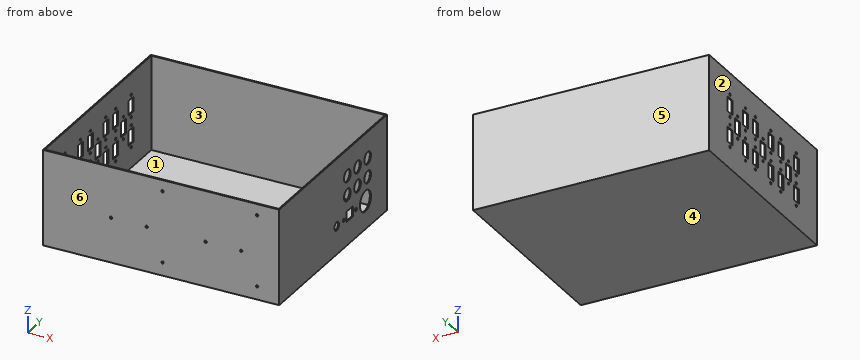
```python
from build123d import *

# Parameters (mm, degrees)
SKETCH2_W                        = 298.45
SKETCH2_H                        = 254
BOSS_EXTRUDE1_DEPTH              = 120.65
SHELL1_T                         = -1.5
PT_CONNECTOR_CUTOUTS_REACH       = 348.06
SKETCH3_R                        = 7.8105
SKETCH3_R_2                      = 2.06375
SKETCH3_R_3                      = 5.334
SKETCH3_R_4                      = 13.0175
SKETCH3_W                        = 13.081
SKETCH3_H                        = 15.748
SKETCH4_R                        = 1.55
SKETCH4_W                        = 18.7
SKETCH4_H                        = 11.8
SOLENOID_CONNECTOR_CUTOUTS_DEPTH = 1.5
SKETCH5_R                        = 1.524
PCB_MOUNTING_HOLES_DEPTH         = 1.5


with BuildPart() as part:
    # Sketch2 → Boss-Extrude1 (new body)
    with BuildSketch(Plane.XY):
        Rectangle(SKETCH2_W, SKETCH2_H)
    extrude(amount=BOSS_EXTRUDE1_DEPTH)

    # Shell1
    shell1_openings = [part.faces().sort_by_distance(p)[0] for p in [
        (0, 0, 120.65),
    ]]
    offset(amount=SHELL1_T, openings=shell1_openings, kind=Kind.INTERSECTION)

    # Sketch3 → PT Connector Cutouts (cut, up to next)
    with BuildSketch(Plane(origin=(149.225, 0, 0), x_dir=(0, 0, -1), z_dir=(1, 0, 0)), mode=Mode.PRIVATE) as pt_connector_cutouts_sk1:
        with Locations((-87.4395, 33.555885142)):
            Circle(SKETCH3_R)
    pt_connector_cutouts_tool1 = extrude(pt_connector_cutouts_sk1.sketch, amount=-PT_CONNECTOR_CUTOUTS_REACH, mode=Mode.PRIVATE) & part.part
    # Sketch3 → PT Connector Cutouts (cut, up to next)
    with BuildSketch(Plane(origin=(149.225, 0, 0), x_dir=(0, 0, -1), z_dir=(1, 0, 0)), mode=Mode.PRIVATE) as pt_connector_cutouts_sk2:
        with Locations((-63.4395, 33.555885142)):
            Circle(SKETCH3_R)
    pt_connector_cutouts_tool2 = extrude(pt_connector_cutouts_sk2.sketch, amount=-PT_CONNECTOR_CUTOUTS_REACH, mode=Mode.PRIVATE) & part.part
    # Sketch3 → PT Connector Cutouts (cut, up to next)
    with BuildSketch(Plane(origin=(149.225, 0, 0), x_dir=(0, 0, -1), z_dir=(1, 0, 0)), mode=Mode.PRIVATE) as pt_connector_cutouts_sk3:
        with Locations((-63.4395, 57.555885142)):
            Circle(SKETCH3_R)
    pt_connector_cutouts_tool3 = extrude(pt_connector_cutouts_sk3.sketch, amount=-PT_CONNECTOR_CUTOUTS_REACH, mode=Mode.PRIVATE) & part.part
    # Sketch3 → PT Connector Cutouts (cut, up to next)
    with BuildSketch(Plane(origin=(149.225, 0, 0), x_dir=(0, 0, -1), z_dir=(1, 0, 0)), mode=Mode.PRIVATE) as pt_connector_cutouts_sk4:
        with Locations((-63.4395, 81.555885142)):
            Circle(SKETCH3_R)
    pt_connector_cutouts_tool4 = extrude(pt_connector_cutouts_sk4.sketch, amount=-PT_CONNECTOR_CUTOUTS_REACH, mode=Mode.PRIVATE) & part.part
    # Sketch3 → PT Connector Cutouts (cut, up to next)
    with BuildSketch(Plane(origin=(149.225, 0, 0), x_dir=(0, 0, -1), z_dir=(1, 0, 0)), mode=Mode.PRIVATE) as pt_connector_cutouts_sk5:
        with Locations((-87.4395, 57.555885142)):
            Circle(SKETCH3_R)
    pt_connector_cutouts_tool5 = extrude(pt_connector_cutouts_sk5.sketch, amount=-PT_CONNECTOR_CUTOUTS_REACH, mode=Mode.PRIVATE) & part.part
    # Sketch3 → PT Connector Cutouts (cut, up to next)
    with BuildSketch(Plane(origin=(149.225, 0, 0), x_dir=(0, 0, -1), z_dir=(1, 0, 0)), mode=Mode.PRIVATE) as pt_connector_cutouts_sk6:
        with Locations((-87.4395, 81.555885142)):
            Circle(SKETCH3_R)
    pt_connector_cutouts_tool6 = extrude(pt_connector_cutouts_sk6.sketch, amount=-PT_CONNECTOR_CUTOUTS_REACH, mode=Mode.PRIVATE) & part.part
    # Sketch3 → PT Connector Cutouts (cut, up to next)
    with BuildSketch(Plane(origin=(149.225, 0, 0), x_dir=(0, 0, -1), z_dir=(1, 0, 0)), mode=Mode.PRIVATE) as pt_connector_cutouts_sk7:
        with Locations((-35.418702679, 25.011064362)):
            Circle(SKETCH3_R_2)
    pt_connector_cutouts_tool7 = extrude(pt_connector_cutouts_sk7.sketch, amount=-PT_CONNECTOR_CUTOUTS_REACH, mode=Mode.PRIVATE) & part.part
    # Sketch3 → PT Connector Cutouts (cut, up to next)
    with BuildSketch(Plane(origin=(149.225, 0, 0), x_dir=(0, 0, -1), z_dir=(1, 0, 0)), mode=Mode.PRIVATE) as pt_connector_cutouts_sk8:
        with Locations(Location((-35.418702679, 53.840064362, 0), (0, 0, 180))):
            Circle(SKETCH3_R_2)
    pt_connector_cutouts_tool8 = extrude(pt_connector_cutouts_sk8.sketch, amount=-PT_CONNECTOR_CUTOUTS_REACH, mode=Mode.PRIVATE) & part.part
    # Sketch3 → PT Connector Cutouts (cut, up to next)
    with BuildSketch(Plane(origin=(149.225, 0, 0), x_dir=(0, 0, -1), z_dir=(1, 0, 0)), mode=Mode.PRIVATE) as pt_connector_cutouts_sk9:
        with Locations((-35.56, 8.501064362)):
            Circle(SKETCH3_R_3)
    pt_connector_cutouts_tool9 = extrude(pt_connector_cutouts_sk9.sketch, amount=-PT_CONNECTOR_CUTOUTS_REACH, mode=Mode.PRIVATE) & part.part
    # Sketch3 → PT Connector Cutouts (cut, up to next)
    with BuildSketch(Plane(origin=(149.225, 0, 0), x_dir=(0, 0, -1), z_dir=(1, 0, 0)), mode=Mode.PRIVATE) as pt_connector_cutouts_sk10:
        with Locations((-35.56, 76.348885142)):
            Circle(SKETCH3_R_4)
    pt_connector_cutouts_tool10 = extrude(pt_connector_cutouts_sk10.sketch, amount=-PT_CONNECTOR_CUTOUTS_REACH, mode=Mode.PRIVATE) & part.part
    # Sketch3 → PT Connector Cutouts (cut, up to next)
    with BuildSketch(Plane(origin=(149.225, 0, 0), x_dir=(0, 0, -1), z_dir=(1, 0, 0)), mode=Mode.PRIVATE) as pt_connector_cutouts_sk11:
        with Locations((-36.546800253, 39.425564362)):
            Rectangle(SKETCH3_W, SKETCH3_H)
    pt_connector_cutouts_tool11 = extrude(pt_connector_cutouts_sk11.sketch, amount=-PT_CONNECTOR_CUTOUTS_REACH, mode=Mode.PRIVATE) & part.part
    add(pt_connector_cutouts_tool1.solids().sort_by_distance((149.225, 33.555885, 87.4395))[0], mode=Mode.SUBTRACT)
    add(pt_connector_cutouts_tool2.solids().sort_by_distance((149.225, 33.555885, 63.4395))[0], mode=Mode.SUBTRACT)
    add(pt_connector_cutouts_tool3.solids().sort_by_distance((149.225, 57.555885, 63.4395))[0], mode=Mode.SUBTRACT)
    add(pt_connector_cutouts_tool4.solids().sort_by_distance((149.225, 81.555885, 63.4395))[0], mode=Mode.SUBTRACT)
    add(pt_connector_cutouts_tool5.solids().sort_by_distance((149.225, 57.555885, 87.4395))[0], mode=Mode.SUBTRACT)
    add(pt_connector_cutouts_tool6.solids().sort_by_distance((149.225, 81.555885, 87.4395))[0], mode=Mode.SUBTRACT)
    add(pt_connector_cutouts_tool7.solids().sort_by_distance((149.225, 25.011064, 35.418703))[0], mode=Mode.SUBTRACT)
    add(pt_connector_cutouts_tool8.solids().sort_by_distance((149.225, 53.840064, 35.418703))[0], mode=Mode.SUBTRACT)
    add(pt_connector_cutouts_tool9.solids().sort_by_distance((149.225, 8.501064, 35.56))[0], mode=Mode.SUBTRACT)
    add(pt_connector_cutouts_tool10.solids().sort_by_distance((149.225, 76.348885, 35.56))[0], mode=Mode.SUBTRACT)
    add(pt_connector_cutouts_tool11.solids().sort_by_distance((149.225, 39.425564, 36.5468))[0], mode=Mode.SUBTRACT)

    # Sketch4 → Solenoid Connector Cutouts (cut)
    with BuildSketch(Plane.ZY.offset(149.225)):
        with Locations(Location((55.387501773, 78.156254231, 0), (0, 0, 270))):
            Circle(SKETCH4_R)
        with Locations(Location((27.162501773, 78.156254231, 0), (0, 0, 90))):
            Circle(SKETCH4_R)
        with Locations(Location((93.487501773, 78.156254231, 0), (0, 0, 270))):
            Circle(SKETCH4_R)
        with Locations(Location((65.262501773, 78.156254231, 0), (0, 0, 90))):
            Circle(SKETCH4_R)
        with Locations(Location((93.487501773, 41.643754231, 0), (0, 0, 270))):
            Circle(SKETCH4_R)
        with Locations(Location((65.262501773, 41.643754231, 0), (0, 0, 90))):
            Circle(SKETCH4_R)
        with Locations(Location((93.487501773, 18.256254231, 0), (0, 0, 270))):
            Circle(SKETCH4_R)
        with Locations(Location((65.262501773, 18.256254231, 0), (0, 0, 90))):
            Circle(SKETCH4_R)
        with Locations(Location((93.487501773, -18.256245769, 0), (0, 0, 270))):
            Circle(SKETCH4_R)
        with Locations(Location((65.262501773, -18.256245769, 0), (0, 0, 90))):
            Circle(SKETCH4_R)
        with Locations(Location((93.487501773, -41.643745769, 0), (0, 0, 270))):
            Circle(SKETCH4_R)
        with Locations(Location((65.262501773, -41.643745769, 0), (0, 0, 90))):
            Circle(SKETCH4_R)
        with Locations(Location((93.487501773, -78.156245769, 0), (0, 0, 270))):
            Circle(SKETCH4_R)
        with Locations(Location((65.262501773, -78.156245769, 0), (0, 0, 90))):
            Circle(SKETCH4_R)
        with Locations(Location((74.437501773, 59.900004231, 0), (0, 0, 270))):
            Circle(SKETCH4_R)
        with Locations(Location((46.212501773, 59.900004231, 0), (0, 0, 90))):
            Circle(SKETCH4_R)
        with Locations(Location((55.387501773, 41.643754231, 0), (0, 0, 270))):
            Circle(SKETCH4_R)
        with Locations(Location((27.162501773, 41.643754231, 0), (0, 0, 90))):
            Circle(SKETCH4_R)
        with Locations(Location((55.387501773, 18.256254231, 0), (0, 0, 270))):
            Circle(SKETCH4_R)
        with Locations(Location((27.162501773, 18.256254231, 0), (0, 0, 90))):
            Circle(SKETCH4_R)
        with Locations(Location((74.437501773, 4.231e-06, 0), (0, 0, 270))):
            Circle(SKETCH4_R)
        with Locations(Location((46.212501773, 4.231e-06, 0), (0, 0, 90))):
            Circle(SKETCH4_R)
        with Locations(Location((55.387501773, -18.256245769, 0), (0, 0, 270))):
            Circle(SKETCH4_R)
        with Locations(Location((27.162501773, -18.256245769, 0), (0, 0, 90))):
            Circle(SKETCH4_R)
        with Locations(Location((55.387501773, -41.643745769, 0), (0, 0, 270))):
            Circle(SKETCH4_R)
        with Locations(Location((27.162501773, -41.643745769, 0), (0, 0, 90))):
            Circle(SKETCH4_R)
        with Locations(Location((74.437501773, -59.899995769, 0), (0, 0, 270))):
            Circle(SKETCH4_R)
        with Locations(Location((46.212501773, -59.899995769, 0), (0, 0, 90))):
            Circle(SKETCH4_R)
        with Locations(Location((55.387501773, -78.156245769, 0), (0, 0, 270))):
            Circle(SKETCH4_R)
        with Locations(Location((27.162501773, -78.156245769, 0), (0, 0, 90))):
            Circle(SKETCH4_R)
        with Locations((41.275001773, 78.156254231)):
            Rectangle(SKETCH4_W, SKETCH4_H)
        with Locations((79.375001773, 78.156254231)):
            Rectangle(SKETCH4_W, SKETCH4_H)
        with Locations((79.375001773, 41.643754231)):
            Rectangle(SKETCH4_W, SKETCH4_H)
        with Locations((79.375001773, 18.256254231)):
            Rectangle(SKETCH4_W, SKETCH4_H)
        with Locations((79.375001773, -18.256245769)):
            Rectangle(SKETCH4_W, SKETCH4_H)
        with Locations((79.375001773, -41.643745769)):
            Rectangle(SKETCH4_W, SKETCH4_H)
        with Locations((79.375001773, -78.156245769)):
            Rectangle(SKETCH4_W, SKETCH4_H)
        with Locations((60.325001773, 59.900004231)):
            Rectangle(SKETCH4_W, SKETCH4_H)
        with Locations((41.275001773, 41.643754231)):
            Rectangle(SKETCH4_W, SKETCH4_H)
        with Locations((41.275001773, 18.256254231)):
            Rectangle(SKETCH4_W, SKETCH4_H)
        with Locations((60.325001773, 4.231e-06)):
            Rectangle(SKETCH4_W, SKETCH4_H)
        with Locations((41.275001773, -18.256245769)):
            Rectangle(SKETCH4_W, SKETCH4_H)
        with Locations((41.275001773, -41.643745769)):
            Rectangle(SKETCH4_W, SKETCH4_H)
        with Locations((60.325001773, -59.899995769)):
            Rectangle(SKETCH4_W, SKETCH4_H)
        with Locations((41.275001773, -78.156245769)):
            Rectangle(SKETCH4_W, SKETCH4_H)
    extrude(amount=-SOLENOID_CONNECTOR_CUTOUTS_DEPTH, mode=Mode.SUBTRACT)

    # Sketch5 → PCB Mounting Holes (cut)
    with BuildSketch(Plane(origin=(0, -127, 127), x_dir=(-1, 0, 0), z_dir=(0, 1, 0))):
        with Locations(Location((-121.235859114, -20.462314931, 0), (0, 0, 270))):
            Circle(SKETCH5_R)
        with Locations(Location((-56.235859114, -70.462314931, 0), (0, 0, 270))):
            Circle(SKETCH5_R)
        with Locations(Location((-121.235859114, -110.462314931, 0), (0, 0, 270))):
            Circle(SKETCH5_R)
        with Locations(Location((-101.235859114, -70.462314931, 0), (0, 0, 270))):
            Circle(SKETCH5_R)
        with Locations(Location((-1.785859114, -20.462314931, 0), (0, 0, 270))):
            Circle(SKETCH5_R)
        with Locations(Location((63.214140886, -70.462314931, 0), (0, 0, 270))):
            Circle(SKETCH5_R)
        with Locations(Location((-1.785859114, -110.462314931, 0), (0, 0, 270))):
            Circle(SKETCH5_R)
        with Locations(Location((18.214140886, -70.462314931, 0), (0, 0, 270))):
            Circle(SKETCH5_R)
    extrude(amount=PCB_MOUNTING_HOLES_DEPTH, mode=Mode.SUBTRACT)


solid = part.part
```
Input: part model. Units: mm. Frame: model coordinates. Face numbers are marked on the shaded views. A direction names the side the tool comes from. Coordinates: 2 decimals unless noted, no trailing zeros. Write each loop counter-clockwise with the first axis right and the second up, starting at its lowest first coordinate (ties: lowest second). Pieces come first, ordered by that corner, then holes.
1) Pin query (flat end, axial travel): pin 1 Ø2.5 at (x, z) = (56.24, 56.54) entering from -Y; pin 2 Ø2 at (x, y) = (-27.5, -74.5) entering from +Z; pin 3 Ø3.5 at (y, z) = (53.84, 35.42) entering from +X (3 decimals). Return the tip coordinate at first contact, or that it passes through.
2) Material intervals for line 1 along X through (y, z) = (3, 83) (3 decimals); line 2 along Y through (x, z) = (-104, 67); line 3 along Z through (x, y) = (-5, -26), sorted ascending.
3) Section A-A on z = 112.5. Output: boundary loops of the cut face in (x, y) (3 decimals).
4) Set-up query: the marked faces 1 and 2. Return all of +Z, -Z, +X, -X, +Y, -Y with unobstructed straight access to the full face (end or side cutting, diameter ignored); none if empty.
5) Mould query, pull axis Y, two halves, no side actions, for the marked faces 3, 4, 5 and 6. Classes: pulls with the +Y half, pulls with the -Y half, needs draft (parallel to the pull), parting line crosses it, or undercut.
6) Section B-B on x = 30. Output: boundary loops of the cut face in (y, z), and give its area (3 significant figures).
Check result:
1. pin 1: stops at y = 125.5
1. pin 2: stops at z = 1.5
1. pin 3: stops at x = -147.725
2. line 1: x = -149.225 to -147.725, 147.725 to 149.225
2. line 2: y = -127 to -125.5, 125.5 to 127
2. line 3: z = 0 to 1.5
3. outline: (-149.225, -127) - (149.225, -127) - (149.225, 127) - (-149.225, 127) - close; hole (-147.725, -125.5) - (147.725, -125.5) - (147.725, 125.5) - (-147.725, 125.5) - close
4. face 1: +Z
4. face 2: +Z, -Z, -X, +Y, -Y
5. face 3: undercut
5. face 4: needs draft
5. face 5: pulls with the +Y half
5. face 6: pulls with the -Y half
6. outline: (-127, 0) - (127, 0) - (127, 120.65) - (125.5, 120.65) - (125.5, 1.5) - (-125.5, 1.5) - (-125.5, 120.65) - (-127, 120.65) - close
6. area: 738 mm2
